Read the model definition and answer for the solid it produces. Units are mm, in the model's axes. Face numbers are marked on the shaded views. A direction names the side the tool comes from. Give positions to 0.01 mm unless a question says otherwise; leave off trailing zeros. Write each loop counter-clockwise with the first axis right and the second up, starting at its lowest first coordinate (ties: lowest second). Pieces come first, ordered by that corner, then holes. Notation, with made-up numbers: (89.5, 51) - (124.5, 51) arc R18 ccw to (124.5, 55) - close; hole circle Ø1 at (2, -36.75). An arc over 180 degrees is marked (long way). Use CSV: the item, a comma, the result in double quotes. Start each with the question number.
from build123d import *

# Parameters (mm, degrees)
F0_R     = 4.7625
F1_DEPTH = 12.7
F2_W     = 10.16
F2_H     = 6.35
F3_DEPTH = 76.2
F4_W     = 6.35
F4_H     = 10.16
F5_DEPTH = 12.7


with BuildPart() as f1:
    # F0 (on Top) → F1 (new body)
    with BuildSketch(Plane.XY):
        with BuildLine():
            Line((-31.75, 44.881477), (-31.75, 25.4))
            Line((-31.75, 25.4), (-19.05, 25.4))
            Line((-19.05, 25.4), (-19.05, 44.881477))
            ThreePointArc((-19.05, 44.881477), (-25.4, 43.18), (-31.75, 44.881477))
        make_face()
        with BuildLine():
            ThreePointArc((-12.7, 55.88), (-31.75, 66.878523), (-31.75, 44.881477))
            ThreePointArc((-31.75, 44.881477), (-25.4, 43.18), (-19.05, 44.881477))
            ThreePointArc((-19.05, 44.881477), (-14.401477, 49.53), (-12.7, 55.88))
        make_face()
        with Locations((-25.4, 55.88)):
            Circle(F0_R, mode=Mode.SUBTRACT)
        Polygon((-50.8, 25.4), (-50.8, 0), (-46.736, 0), (-46.736, 19.05), (-29.464, 19.05), (-29.464, 0), (-21.336, 0), (-21.336, 19.05), (-4.064, 19.05), (-4.064, 0), (0, 0), (0, 25.4), (-19.05, 25.4), (-31.75, 25.4), align=None)
    extrude(amount=F1_DEPTH)

    # F2 (on face) → F3 (join)
    with BuildSketch(Plane.YZ):
        with Locations((12.7, 3.175)):
            Rectangle(F2_W, F2_H)
    extrude(amount=F3_DEPTH)

    # F4 (on face) → F5 (join)
    with BuildSketch(Plane.XY.offset(6.35)):
        with Locations((73.025, 12.7)):
            Rectangle(F4_W, F4_H)
    extrude(amount=F5_DEPTH)


solid = f1.part
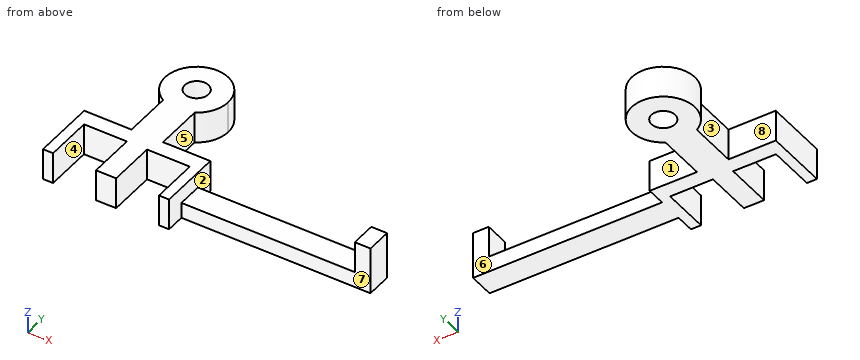
(1) The part is cut by section C-C on y = 31.5. Write down the section's boundary in (x, z), plus the area to 3 significant figures.
(2) Consider probe 1 along X at (y, z) = (12, 10); probe 2 along X at (y, z) = (4.5, 7.75); probe 3 along Y at (x, z) = (-25.4, 4.75). Determine where each line is inside the solid, lowest interval first.
(3) The part is cut by section A-A on z = 8. Give the number of separate pieces and of enclosed holes in the cut face, plus the area to 3 significant figures.
(4) Which of the six approach directions +Z, -Z, +X, -X, +Y, -Y give full straight-line access (tool end or side, diameter ignored) to the marked faces 4, 5, 6, 7 and 8?
(5) Given P1, Ø6.5, axis at y = 37, z = 6, coming from the -X side; P2, Ø3, axis at y = 51, z = 6, coming from the +X side; P3, Ø4, axis at x = -41.5, z = 3.5, coming from the +Y side, each flat-ended and moving along its own axis, determine where each tip first touches the part or whether it passes through.
(6) The part is cut by section B-B on x = -25.4. Write down the section's boundary in (y, z), plus the area to 3 significant figures.
(7) For a pull along X with two mould halves and no side action, classify the marked faces 1, 2 and 3 as pulls with the +X half, pulls with the -X half, needs draft (parallel to the pull), parting line crosses it, or undercut.
(8) The part is cut by section D-D on z = 15. Write down the section's boundary in (x, y).
Reported:
1,outline,"(-31.75, 0) - (-19.05, 0) - (-19.05, 12.7) - (-31.75, 12.7) - close"
1,area,"161 mm²"
2,probe 1,"-50.8 to -46.74, -29.46 to -21.34, -4.06 to 0, 69.85 to 76.2"
2,probe 2,"-50.8 to -46.74, -29.46 to -21.34, -4.06 to 0"
2,probe 3,"0 to 51.12, 60.64 to 68.58"
3,separate pieces,"2"
3,enclosed holes,"1"
3,area,"1,370 mm²"
4,face 4,"+Z, -Z, -Y"
4,face 5,"+Z, -Z, +X"
4,face 6,"+Z, -Z, +X, +Y"
4,face 7,"+Z, -Z, +X, -Y"
4,face 8,"+Z, -Z, -X"
5,P1,"x = -31.75"
5,P2,"x = -13.16"
5,P3,"y = 25.4"
6,outline,"(0, 0) - (51.12, 0) - (51.12, 12.7) - (0, 12.7) - close; (60.64, 0) - (68.58, 0) - (68.58, 12.7) - (60.64, 12.7) - close"
6,area,"750 mm²"
7,face 1,"needs draft"
7,face 2,"undercut"
7,face 3,"pulls with the -X half"
8,outline,"(69.85, 7.62) - (76.2, 7.62) - (76.2, 17.78) - (69.85, 17.78) - close"
